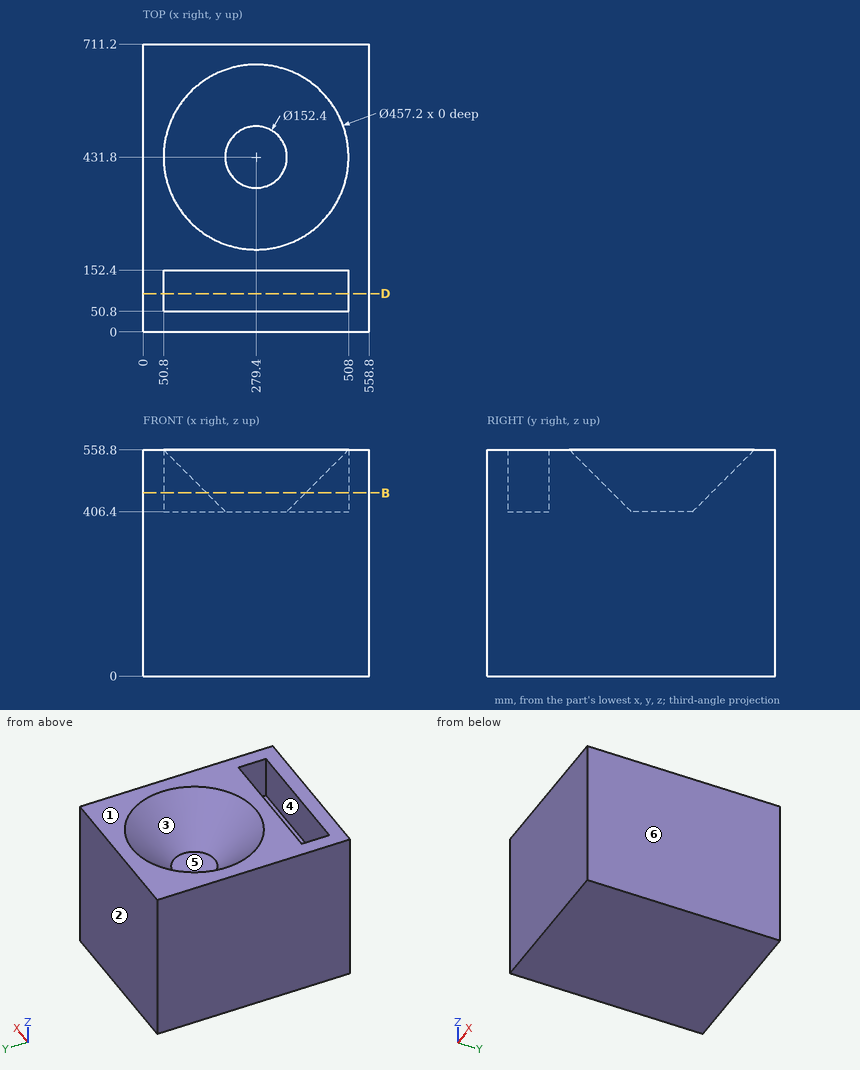
Geometry check sheet. Reference: drawing and pictorial views, mm from the part's lowest x, y, z. A direction names the side the tool comes from. Give positions to 0.01 mm unless a question says otherwise; leave off trailing zeros. Loops run counter-clockwise (first coordinate to the right, second up) from the corner with the lowest first, then second, coordinate; pieces in that order, holes last. Notation, with made-up numbers: M -16,-16 L 30,-16 A24 ccw 30,-4 Z; hole C 38.5,-23.5 d2. An arc over 180 degrees is marked long. One line per question, with ' | ' between items.
Item 1: Tool access check on the marked faces 5 and 6. Record the directions out of +Z, -Z, +X, -X, +Y, -Y that give a thin tool (end or side, any length) a straight path to the whole face; none if there is none.
Completed:
face 5: +Z | face 6: +Z, -Z, +X, +Y, -Y
Item 2: Section check B-B, the plane z = 452.5. Record the cut outline in (x, y), plus the area to 3 significant figures.
Completed:
outline: M 0,0 L 558.8,0 L 558.8,711.2 L 0,711.2 Z; hole M 50.8,50.8 L 508,50.8 L 508,152.4 L 50.8,152.4 Z; hole C 279.4,431.8 d244.6 | area: 304,000 mm^2
Item 3: Draft check along Y on the marked faces 1, 2, 3 and 4. Enter one of: +Y half, -Y half, draft (parallel to the pull), parting line (faces both ways), or undercut.
Completed:
face 1: draft | face 2: +Y half | face 3: undercut | face 4: undercut
Item 4: Section check D-D, the plane y = 94.5. Record the cut outline in (x, z).
Completed:
outline: M 0,0 L 558.8,0 L 558.8,558.8 L 508,558.8 L 508,406.4 L 50.8,406.4 L 50.8,558.8 L 0,558.8 Z
Item 5: Thickness scan on line 1 (Y direction, x = 411, z = 482); line 2 (Y direction, x = 279, z = 558); line 3 (Y direction, x = 420, z = 420). Record the ranges inside material, lowest first. Write a range as [from, to].
Completed:
line 1: y = [0, 50.8], [152.4, 356.14], [507.46, 711.2] | line 2: y = [0, 50.8], [152.4, 204], [659.6, 711.2] | line 3: y = [0, 50.8], [152.4, 711.2]
Item 6: Depth check by flat-ended pin: P1, Ø1.5, axis at x = 348.5, y = 450, coming from the +Z side; P2, Ø12, axis at x = 114, y = 419.5, coming from the +Z side; P3, Ø4, axis at x = 457.5, y = 346.5, coming from the +Z side. Enter the tip coordinate at first touch or a pass-through.
Completed:
P1: stops at z = 406.4 | P2: stops at z = 502.06 | P3: stops at z = 529.67
